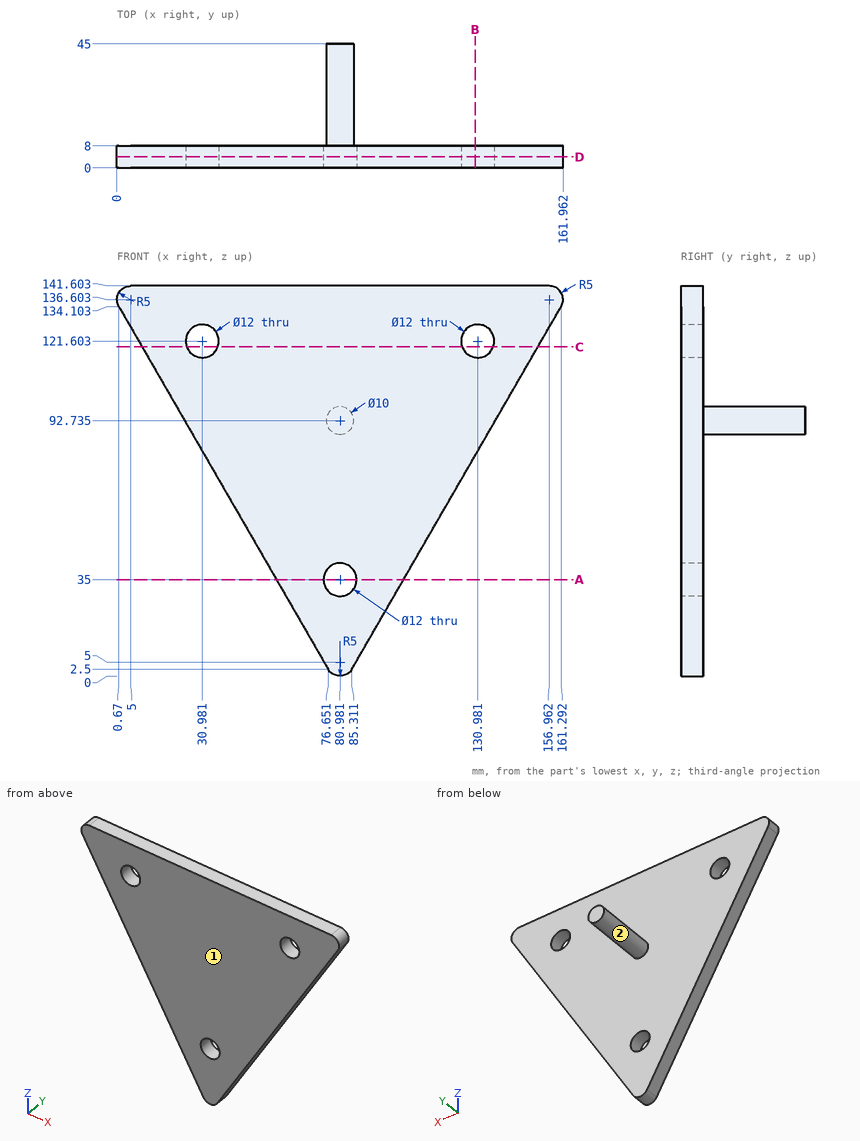
The drawing under review shows one solid part. Ordinate dimensions are in mm from its lowest x, y, z. A direction names the side the tool comes from. Coordinates: 2 decimals unless noted, no trailing zeros. Order: outer loops, then holes, each group sorted by start corner. A loop starts at its lowest first (then second) coordinate and runs counter-clockwise, first axis right, second up. Notation, with made-up numbers: (69, -29.75) -> (76, -29.75) arc R24 ccw to (76, -17.75) -> close; hole circle Ø2 at (71, 2). An arc over 180 degrees is marked (long way). Answer in a Markdown table with one row per item.
(1) Machinability: for the marked faces 1 and 2, which of the approach directions +Z, -Z, +X, -X, +Y, -Y give a long, thin tool a straight path to every point of the face, cutting with its end or side? Answer none if there is none.
Answers:
| item | result |
|---|---|
| face 1 | +Z, -Z, +X, -X, -Y |
| face 2 | +Y |
(2) Wall thickness on line 1 along X through (y, z) = (5, 120); line 2 along Y through (x, z) = (62, 98); line 3 along X through (y, z) = (7.5, 37.5) (1 decimal): over which ranges is each line inside the solid? List them lowest first.
Answers:
| item | result |
|---|---|
| line 1 | 8.81 to 25.2, 36.76 to 125.2, 136.76 to 153.15 |
| line 2 | 0 to 8 |
| line 3 | 56.4 to 75.5, 86.4 to 105.5 |
(3) Consider section A-A (z = 35). Write out the cut boundary in (x, y) (1 decimal).
Answers:
| item | result |
|---|---|
| outline | (57.9, 0) -> (75, 0) -> (75, 8) -> (57.9, 8) -> close; (87, 0) -> (104.1, 0) -> (104.1, 8) -> (87, 8) -> close |
(4) Consider section C-C (z = 119.5). Write out the cut boundary in (x, y).
Answers:
| item | result |
|---|---|
| outline | (9.1, 0) -> (25.36, 0) -> (25.36, 8) -> (9.1, 8) -> close; (36.6, 0) -> (125.36, 0) -> (125.36, 8) -> (36.6, 8) -> close; (136.6, 0) -> (152.86, 0) -> (152.86, 8) -> (136.6, 8) -> close |
(5) Insertion check: pin 1 (2 mm diameter, centred on x = 78, z = 49.5, fed in from +Y); pin 2 (7 mm diameter, centred on x = 80.98, z = 35, fed in from -Y). Each pin has a flat end and moves straight along its axis. Give the tip position at first contact, or say it passes through.
Answers:
| item | result |
|---|---|
| pin 1 | y = 8 |
| pin 2 | through |
(6) Consider section B-B (x = 130). Write out the cut boundary in (y, z), plus the area to 3 significant figures.
Answers:
| item | result |
|---|---|
| outline | (0, 79.9) -> (8, 79.9) -> (8, 115.68) -> (0, 115.68) -> close; (0, 127.52) -> (8, 127.52) -> (8, 141.6) -> (0, 141.6) -> close |
| area | 399 mm² |
(7) Consider section D-D (y = 4). Write out the cut boundary in (x, z), plus the area to 3 significant figures.
Answers:
| item | result |
|---|---|
| outline | (0.67, 134.1) -> (76.65, 2.5) arc R5 ccw to (85.31, 2.5) -> (161.29, 134.1) arc R5 ccw to (156.96, 141.6) -> (5, 141.6) arc R5 ccw to start; hole circle Ø12 at (30.98, 121.6); hole circle Ø12 at (80.98, 35); hole circle Ø12 at (130.98, 121.6) |
| area | 12,000 mm² |
